Here's how the part is built. I have some questions about the finished solid (model axes, mm). Face numbers are marked on the shaded views. A direction names the side the tool comes from. Give positions to 0.01 mm unless a question says otherwise; leave off trailing zeros. Write each loop counter-clockwise with the first axis right and the second up, starting at its lowest first coordinate (ties: lowest second). Pieces come first, ordered by that corner, then holes. Notation, with made-up numbers: M 69,-16.5 L 103,-16.5 A22 cw 103,1.5 Z; hole C 61.25,-38 d11. An arc over 180 degrees is marked long. Use one line per item in the form item = value. Start each with the question number.
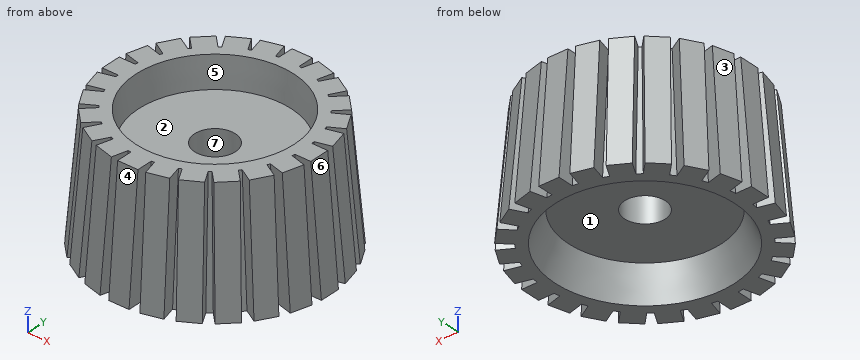
from build123d import *

# Parameters (mm, degrees)
F3_DEPTH      = 1
F3_DEPTH_BACK = 1
F4_COUNT      = 24
F4_ANGLE      = 345
F5_R          = 2
F6_DEPTH      = 25


with BuildPart() as f1:
    # F0 (on Front) → F1 (revolve)
    with BuildSketch(Plane.XZ):
        Polygon((7.5, 0), (0, 0), (0, -6), (7.5, -6), (8.8123299529, -9), (9.8123299529, -9), (8.7624659906, 3), (7.7624659906, 3), align=None)
    revolve(axis=Axis((0, 0, -3), (0, 0, 1)))

    # F2 (on Front) → F3 (join, two sides)
    with BuildSketch(Plane.XZ) as f3_sk:
        Polygon((10.2624659906, 3), (8.7624659906, 3), (7.7624659906, 3), (8.8123299529, -9), (9.8123299529, -9), (11.3123299529, -9), align=None)
    extrude(amount=F3_DEPTH)
    extrude(f3_sk.sketch, amount=-F3_DEPTH_BACK)

    # F4: F1 ×24 about axis
    f4_axis = Axis((0, 0, 3), (0, 0, 1))


with BuildPart() as f1_1:
    add(f1.part)
    for i in range(1, F4_COUNT):
        add(f1.part.rotate(f4_axis, i * F4_ANGLE / (F4_COUNT - 1)))

    # F5 (on face) → F6 (cut)
    with BuildSketch(Plane.XY):
        Circle(F5_R)
    extrude(amount=-F6_DEPTH, mode=Mode.SUBTRACT)


solid = f1_1.part
1) Please list where these lines run through material, in increasing order: line 1 (Y direction, x = 0, z = -2.95); line 2 (X direction, y = 6, z = 1); line 3 (X direction, y = -0.75, z = -4.5).
2) On a 3-axis mill with a long thin cutter (end or side, diameter ignored), from which of +Z, -Z, +X, -X, +Y, -Y can I reach the whole of each face in a straight line? I mean the marked faces 1, 2 and 3. Say none if no direction works.
3) Suppose I cut it at A-A, the plane y = 0. List the corners of the cut face in (x, z) for me.
4) Will these pins go through, and if not, where does the flat tip stop? P1, Ø6, axis at y = 8, z = -6.5, coming from the +X side; P2, Ø1.3, axis at y = 10.5, z = -0.5, coming from the -X side; P3, Ø4.5, axis at x = -0.5, y = 0, coming from the -Z side.
5) Thinking about a two-plate mould opening in Y: for the marked faces 4, 5, 6 and 7, which applies, released by +Y, released by -Y, zero draft, split by the parting line, or undercut?
Checks:
q1.line_1 = -10.78 to -2, 2 to 10.78
q1.line_2 = -8.59 to -8.39, -7.41 to -4.64, 4.64 to 7.41, 8.39 to 8.59
q1.line_3 = -10.92 to -1.85, 1.85 to 10.92
q2.face_1 = -Z
q2.face_2 = +Z
q2.face_3 = +Z, -X, +Y
q3.outline = M -11.31,-9 L -8.81,-9 L -7.5,-6 L -2,-6 L -2,0 L -7.5,0 L -7.76,3 L -10.26,3 Z; M 2,-6 L 7.5,-6 L 8.81,-9 L 11.31,-9 L 10.26,3 L 7.76,3 L 7.5,0 L 2,0 Z
q4.P1 = 9.95
q4.P2 = -3.71
q4.P3 = -6
q5.face_4 = released by -Y
q5.face_5 = undercut
q5.face_6 = zero draft
q5.face_7 = undercut
